Build history of the part. All positions in model axes, mm. Face numbers are marked on the shaded views. Round coordinates to 2 decimals unless told otherwise and drop trailing zeros. Order: outer loops, then holes, each group sorted by start corner. A loop starts at its lowest first (then second) coordinate and runs counter-clockwise, first axis right, second up. Notation, with made-up numbers: (-11, 26) -> (18, 26) arc R17 ccw to (18, 35) -> close; hole circle Ø11 at (-39, -6). An arc over 180 degrees is marked (long way). Answer as a JSON object with one key per item and string values.
from build123d import *

# Parameters (mm, degrees)
ESQUISSE1_R        = 5
ESQUISSE1_R_2      = 1.75
BOSS_EXTRU_1_DEPTH = 2
BOSS_EXTRU_2_DEPTH = 2
CONG_1_R           = 2


with BuildPart() as part:
    # Esquisse1 → Boss.-Extru.1 (new body)
    with BuildSketch(Plane.XY):
        Circle(ESQUISSE1_R)
        Circle(ESQUISSE1_R_2, mode=Mode.SUBTRACT)
    extrude(amount=BOSS_EXTRU_1_DEPTH)

    # Esquisse2 → Boss.-Extru.2 (add)
    with BuildSketch(Plane.XY.offset(2)):
        Polygon((10, 7.5), (10, -7.5), (2, -4.582575695), (2, 4.582575695), align=None)
    extrude(amount=-BOSS_EXTRU_2_DEPTH)

    # Congé1
    cong_1_edges = [part.edges().sort_by_distance(p)[0] for p in [
        (2, 4.582575695, 1),
        (10, 7.5, 1),
        (10, -7.5, 1),
        (2, -4.582575695, 1),
    ]]
    fillet(cong_1_edges, radius=CONG_1_R)


solid = part.part
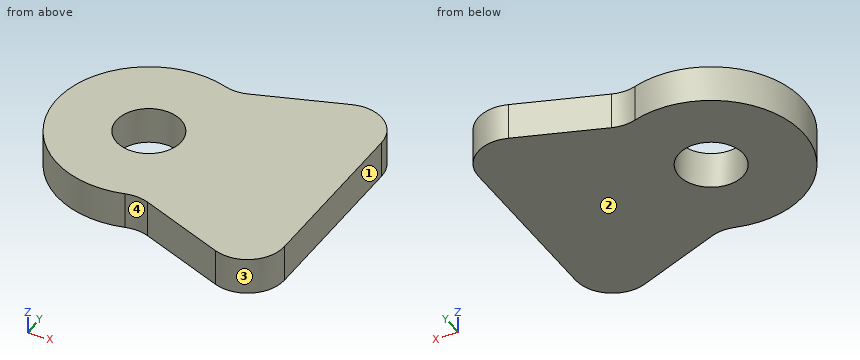
1) Cut at C-C, the plane z = 0.75. Give the cut face in (x, y), plus the area to 3 significant figures.
Checked values:
{"outline": "(1.43, -4.79) arc R2 cw to (2.68, -4.83) -> (7.31, -6.52) arc R2 ccw to (10, -4.64) -> (10, 4.64) arc R2 ccw to (7.31, 6.52) -> (2.68, 4.83) arc R2 cw to (1.43, 4.79) arc R5 ccw (long way) to start; hole circle Ø3.5 at (0, 0)", "area": "142 mm²"}
2) Probe L1, parallel to Y at x = 0, z = 1.2; L2, parallel to Y at x = -1.5, z = 1.3; L3, parallel to X at y = -4.5, z = 0.25. List the from-to ranges inside material, lowest first. Write a range as from..to.
Checked values:
{"L1": "y = -5..-1.75, 1.75..5", "L2": "y = -4.77..-0.9, 0.9..4.77", "L3": "x = -2.18..10"}
3) Cut at A-A, the plane x = 0. Give the cut face in (y, z).
Checked values:
{"outline": "(-5, 0) -> (-1.75, 0) -> (-1.75, 2) -> (-5, 2) -> close; (1.75, 0) -> (5, 0) -> (5, 2) -> (1.75, 2) -> close"}
4) Pull direction X, two halves, no side cores. Call the marked faces 1, 2, 3 and 4: pulls with the +X half, pulls with the -X half, needs draft (parallel to the pull), parting line crosses it, or undercut.
Checked values:
{"face 1": "pulls with the +X half", "face 2": "needs draft", "face 3": "parting line crosses it", "face 4": "undercut"}
5) Cut at B-B, the plane y = 0. Give the cut face in (x, z), plus the area to 3 significant figures.
Checked values:
{"outline": "(-5, 0) -> (-1.75, 0) -> (-1.75, 2) -> (-5, 2) -> close; (1.75, 0) -> (10, 0) -> (10, 2) -> (1.75, 2) -> close", "area": "23.0 mm²"}
6) Cut at D-D, the plane y = -3.5. Give the cut face in (x, z), plus the area to 3 significant figures.
Checked values:
{"outline": "(-3.57, 0) -> (10, 0) -> (10, 2) -> (-3.57, 2) -> close", "area": "27.1 mm²"}
7) Flat gauge pin, fed straight in: pin 1 Ø2 at (x, y) = (0, 0) entering from +Z. Where does the tip first touch, or does it go through?
Checked values:
{"pin 1": "passes through"}
